Could you check a few things on this model? Use its own coordinates, in mm. A direction names the side the tool comes from. Give positions to 0.01 mm unless a question says otherwise; leave off trailing zeros. Loops run counter-clockwise (first coordinate to the right, second up) from the corner with the lowest first, then second, coordinate; pieces in that order, holes last. Notation, with made-up numbers: (70.5, 20.25) -> (103.5, 20.25) arc R26 ccw to (103.5, 50.25) -> close; hole circle Ø10 at (10.5, 66). An arc over 180 degrees is marked (long way). Write item = value, one per line. Start each with the question number.
1) I'm going to push flat-ended pins straight in: pin 1 Ø1 at (x, z) = (0.5, 16) entering from -Y (3 decimals); pin 2 Ø2 at (y, z) = (3, -17) entering from -X; pin 3 Ø2 at (y, z) = (1, -20.5) entering from +X (3 decimals); pin 4 Ø1.4 at (y, z) = (-0.5, 37) entering from -X. Where does each tip first touch, or does it pass through?
2) I need wall thicknesses on probe 1 along Z at (x, y) = (-0.25, 0) (3 decimals); probe 2 along Z at (x, y) = (0, -4.5); probe 3 along Y at (x, z) = (0, -18.5) (3 decimals). Which ranges of each line are inside material? Lowest first, please. Write a range as from..to.
3) If we mould it in two halves opening along X, with no side actions, what happens to faces 4 (the face through (1.03, 4.65, 34.97)), 5 (the face through (1.21, 2.05, 36.45)), 6 (the face through (0, 0, -38.1)), 7 (the face through (-1.21, -2.05, 36.45))? For each: +X half, -X half, draft (parallel to the pull), parting line (faces both ways), or undercut.
4) On a 3-axis mill with a long thin cutter (end or side, diameter ignored), from which of +Z, -Z, +X, -X, +Y, -Y can I reach the whole of each face in a straight line? I mean faces 1 (the face through (2.52, 1.93, -2.22)), 2 (the face through (1.174, -2.072, 36.452)), 3 (the face through (-2, 3, 38.1)). Say none if no direction works.
5) I want a section at B-B (z = 21). List the corners of the cut face in (x, y) for me (3 decimals), and give its area (3 significant figures).
from build123d import *

# Parameters (mm, degrees)
CUT_EXTRUDE1_START = 38.1
CUT_EXTRUDE1_DEPTH = 3.175


with BuildPart() as part:
    # Sketch2 → Revolve1 (revolve)
    with BuildSketch(Plane(origin=(0, 0, 0), x_dir=(0, 0, -1), z_dir=(1, 0, 0)), mode=Mode.PRIVATE) as revolve1_sk:
        with BuildLine():
            Line((38.1, 0), (38.1, 2.2225))
            Line((38.1, 2.2225), (37.1475, 3.175))
            Line((37.1475, 3.175), (-31.75, 3.175))
            Line((-31.75, 3.175), (-31.75, 4.445))
            ThreePointArc((-31.75, 4.445), (-31.842993597, 4.669506403), (-32.0675, 4.7625))
            Line((-32.0675, 4.7625), (-37.7825, 4.7625))
            ThreePointArc((-37.7825, 4.7625), (-38.007006403, 4.669506403), (-38.1, 4.445))
            Line((-38.1, 4.445), (-38.1, 0))
            Line((-38.1, 0), (38.1, 0))
        make_face()
    revolve(revolve1_sk.sketch.rotate(Axis((0, 0, -38.1), (0, 0, 1)), 90), axis=Axis((0, 0, -38.1), (0, 0, 1)))

    # Sketch3 → Cut-Extrude1 (cut)
    with BuildSketch(Plane.XY.offset(CUT_EXTRUDE1_START)):
        Polygon((-2.38125, 1.374815329), (-2.38125, -1.374815329), (0, -2.749630657), (2.38125, -1.374815329), (2.38125, 1.374815329), (0, 2.749630657), align=None)
    extrude(amount=-CUT_EXTRUDE1_DEPTH, mode=Mode.SUBTRACT)

    # Cut-Extrude2 cone 1 section (through the dimple's axis) → Cut-Extrude2 (revolve, cut)
    with BuildSketch(Plane(origin=(0, 0, 38.1), x_dir=(0, -1, 0), z_dir=(1, 0, 0))):
        Polygon((0, 0), (3.032192214, 0), (0, 1.750636991), align=None)
    revolve(axis=Axis((0, 0, 38.1), (0, 0, -1)), mode=Mode.SUBTRACT)


solid = part.part
Answer list:
q1.pin_1 = -3.175
q1.pin_2 = -2.47
q1.pin_3 = 3.175
q1.pin_4 = -4.76
q2.probe_1 = -38.1..34.925
q2.probe_2 = 31.75..38.1
q2.probe_3 = -3.175..3.175
q3.face_4 = parting line
q3.face_5 = undercut
q3.face_6 = draft
q3.face_7 = undercut
q4.face_1 = -Z
q4.face_2 = +Z
q4.face_3 = +Z, +X, -X, +Y, -Y
q5.outline = circle Ø6.35 at (0, 0)
q5.area = 31.7 mm^2
